```python
from build123d import *

# Parameters (mm, degrees)
SKETCH1_R           = 20
BASE_EXTRUDE_DEPTH  = 425
SKETCH4_R           = 7.5
BOSS_EXTRUDE1_DEPTH = 6.25


with BuildPart() as part:
    # Sketch1 → Base-Extrude (new body)
    with BuildSketch(Plane.XY):
        Circle(SKETCH1_R)
    extrude(amount=-BASE_EXTRUDE_DEPTH)

    # Sketch4 → Boss-Extrude1 (add, symmetric)
    with BuildSketch(Plane(origin=(0, 0, 0), x_dir=(-1, 0, 0), z_dir=(0, 1, 0))):
        with BuildLine():
            Line((-19, -60), (-19, 0))
            ThreePointArc((-19, 0), (-49, -30), (-19, -60))
        make_face()
        with Locations(Location((-37, -30, 0), (0, 0, 90))):
            Circle(SKETCH4_R, mode=Mode.SUBTRACT)
    extrude(amount=BOSS_EXTRUDE1_DEPTH, both=True)


solid = part.part
```
Work out the finished part from the listing and answer in its coordinate system (mm). A direction names the side the tool comes from. Coordinates: 2 decimals unless noted, no trailing zeros. Order: outer loops, then holes, each group sorted by start corner. A loop starts at its lowest first (then second) coordinate and runs counter-clockwise, first axis right, second up. Notation, with made-up numbers: M -33.75,-3.75 L -16.75,-3.75 A10 cw -16.75,2.25 Z; hole C 72.25,49.25 d10. An arc over 180 degrees is marked long. Use CSV: the item, a comma, the result in double quotes.
1) Section D-D on z = -147 is taken. Write down the section's boundary in (x, y).
Worked out:
outline,"C 0,0 d40"
2) Flat-ended cylindrical pins translate along their axes: pin 1 Ø1 at (x, y) = (17.5, -5.5) entering from +Z; pin 2 Ø4 at (y, z) = (-5.5, -89) entering from -X; pin 3 Ø8 at (y, z) = (10, -111.5) entering from -X; pin 4 Ø13.5 at (x, z) = (37, -30) entering from +Y. Find the tip coordinate at first contact, or state that the pin passes through.
Worked out:
pin 1,"stops at z = 0"
pin 2,"stops at x = -19.69"
pin 3,"stops at x = -19.08"
pin 4,"passes through"
3) For faces 1 (the face through (28, -6.25, -30)), 2 (the face through (28, 6.25, -30)), 3 (the face through (0, 0, -425)), determine the directions among +Z, -Z, +X, -X, +Y, -Y from which every point of the face is accessible in a straight line to the end or side of a thin tool.
Worked out:
face 1,"+Z, -Z, +X, -Y"
face 2,"+Z, -Z, +X, +Y"
face 3,"-Z, +X, -X, +Y, -Y"
4) Section A-A on z = -30 is taken. Write down the section's boundary in (x, y) (3 decimals), plus the area to 3 significant figures.
Worked out:
outline,"M 19,-6.25 L 29.5,-6.25 L 29.5,6.25 L 19,6.25 L 19,6.245 A20 ccw long 19,-6.245 Z; M 44.5,-6.25 L 49,-6.25 L 49,6.25 L 44.5,6.25 Z"
area,"1,440 mm^2"
5) Section B-B on x = 37 is taken. Write down the section's boundary in (y, z), plus the area to 4 significant figures.
Worked out:
outline,"M -6.25,-54 L 6.25,-54 L 6.25,-37.5 L -6.25,-37.5 Z; M -6.25,-22.5 L 6.25,-22.5 L 6.25,-6 L -6.25,-6 Z"
area,"412.5 mm^2"
6) Determine the mould class of faces 4 (the face through (48.993, 0.088, -29.34)), 5 (the face through (-16, -12, -210)), 6 (the face through (0, 0, 0)), 7 (the face through (29.68, -0.09, -31.63)) for opening direction X: released by +X, released by -X, zero draft, split by the parting line, or undercut.
Worked out:
face 4,"released by +X"
face 5,"split by the parting line"
face 6,"zero draft"
face 7,"undercut"
7) Consider line 1 (X direction, y = -1.75, z = -30); line 2 (X direction, y = 0, z = -30); line 3 (Y direction, x = -1, z = -196). Determine where each line is inside the solid, lowest interval first. Write a range as [from, to].
Worked out:
line 1,"x = [-19.92, 29.5], [44.5, 49]"
line 2,"x = [-20, 29.5], [44.5, 49]"
line 3,"y = [-19.97, 19.97]"
